Part model, mm, in its own coordinate system. Face numbers are marked on the shaded views. A direction names the side the tool comes from. Coordinates: 2 decimals unless noted, no trailing zeros. Loops run counter-clockwise (first coordinate to the right, second up) from the corner with the lowest first, then second, coordinate; pieces in that order, holes last. Notation, with made-up numbers: (-21.75, 29) -> (-17.75, 29) arc R27 ccw to (-17.75, 48) -> close; hole circle Ø10 at (43, -27). An arc over 180 degrees is marked (long way). Use one line per item in the form item = value. Start each with the question number.
(1) Mould opens along Y. For the marked faces 3, 4, 5 and 6 say: +Y half, -Y half, draft (parallel to the pull), parting line (faces both ways), or undercut.
(2) Band-saw the part on D-D on y = -6. Count the separate pieces of the cut face and the enclosed holes in it, then the cut area to 3 significant figures.
(3) Band-saw the part on A-A on x = 0. Give the cut face in (y, z).
(4) Band-saw the part on B-B on z = -1. Give the cut face in (x, y).
(5) Drill centre lines: L1, parallel to Z at x = -1, y = 0.5; L2, parallel to Z at x = -20, y = 1.75; L3, parallel to Y at x = -21, z = -10.5. Where is each one in solid material? Low to high. Write a range as [from, to].
(6) 3-axis set-ups, long thin cutter, end or side, ignore diameter. For the marked faces 1 and 2: which of +Z, -Z, +X, -X, +Y, -Y reach the whole face in a straight line?
(7) Band-saw the part on C-C on x = -27. Give the cut face in (y, z).
(8) Pin check, flat tips, straight feed: P1, Ø2, axis at x = 0, y = -6, coming from the -Z side; P2, Ø1.7, axis at x = -9.88, y = -6, coming from the -Z side; P3, Ø0.6, axis at y = 0.5, z = -8.5, coming from the -X side; P4, Ø2.5, axis at y = 0, z = 13, coming from the +X side. Stop position of each tip, or through.
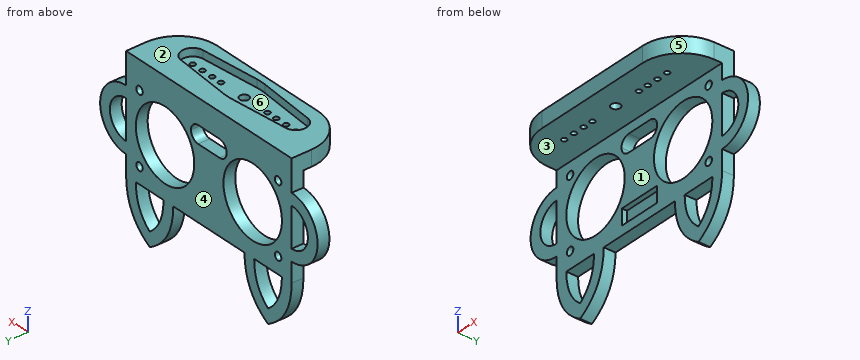
```python
from build123d import *

# Parameters (mm, degrees)
SKETCH1_R           = 1
SKETCH1_R_2         = 9
BOSS_EXTRUDE3_DEPTH = 3
BOSS_EXTRUDE4_DEPTH = 15
SKETCH5_R           = 0.6604
SKETCH5_R_2         = 1.143
CUT_EXTRUDE1_DEPTH  = 10
FILLET2_R           = 10
CUT_EXTRUDE3_DEPTH  = 2
SKETCH8_W           = 10.76
SKETCH8_H           = 4
CUT_EXTRUDE4_DEPTH  = 1.3


with BuildPart() as part:
    # Sketch1 → Boss-Extrude3 (new body)
    with BuildSketch(Plane(origin=(0, 0, 0), x_dir=(1, 0, 0), z_dir=(0, 1, 0))):
        with BuildLine():
            Line((-25.5, -8), (-25.5, -13))
            Line((-25.5, -13), (25.5, -13))
            Line((25.5, -13), (25.5, -8))
            ThreePointArc((25.5, -8), (33.5, 0), (25.5, 8))
            Line((25.5, 8), (25.5, 13))
            add(Edge.make_bspline(
                [(25.5, 13), (25.447957122, 21.830633136), (18.232464907, 26.037260317)],
                knots=[0, 0, 0, 1, 1, 1], degree=2))
            add(Edge.make_bspline(
                [(10.964929815, 13), (11.016972693, 21.830633136), (18.232464907, 26.037260317)],
                knots=[0, 0, 0, 1, 1, 1], degree=2))
            Line((10.964929815, 13), (-10.964929815, 13))
            add(Edge.make_bspline(
                [(-10.964929815, 13), (-11.016972693, 21.830633136), (-18.232464907, 26.037260317)],
                knots=[0, 0, 0, 1, 1, 1], degree=2))
            add(Edge.make_bspline(
                [(-25.5, 13), (-25.447957122, 21.830633136), (-18.232464907, 26.037260317)],
                knots=[0, 0, 0, 1, 1, 1], degree=2))
            Line((-25.5, 13), (-25.5, 8))
            ThreePointArc((-25.5, 8), (-33.5, 0), (-25.5, -8))
        make_face()
        with Locations((-21.330701069, -8.788977071)):
            Circle(SKETCH1_R, mode=Mode.SUBTRACT)
        with BuildLine():
            ThreePointArc((-25.5, -5), (-30.5, 0), (-25.5, 5))
            Line((-25.5, 5), (-25.5, -5))
        make_face(mode=Mode.SUBTRACT)
        with Locations((-13.5, 0)):
            Circle(SKETCH1_R_2, mode=Mode.SUBTRACT)
        with BuildLine():
            ThreePointArc((-5.5, -7.45), (-4.855634919, -5.894365081), (-3.3, -5.25))
            Line((-3.3, -5.25), (3.3, -5.25))
            ThreePointArc((3.3, -5.25), (4.855634919, -5.894365081), (5.5, -7.45))
            ThreePointArc((5.5, -7.45), (4.855634919, -9.005634919), (3.3, -9.65))
            Line((3.3, -9.65), (-3.3, -9.65))
            ThreePointArc((-3.3, -9.65), (-4.855634919, -9.005634919), (-5.5, -7.45))
        make_face(mode=Mode.SUBTRACT)
        with Locations((21.36922293, -8.864067488)):
            Circle(SKETCH1_R, mode=Mode.SUBTRACT)
        with Locations((13.5, 0)):
            Circle(SKETCH1_R_2, mode=Mode.SUBTRACT)
        with BuildLine():
            Line((25.5, -5), (25.5, 5))
            ThreePointArc((25.5, 5), (30.5, 0), (25.5, -5))
        make_face(mode=Mode.SUBTRACT)
        with Locations((-21.330701069, 8.788977071)):
            Circle(SKETCH1_R, mode=Mode.SUBTRACT)
        with BuildLine():
            add(Edge.make_bspline(
                [(-18.232464907, 22.430397358), (-17.881752173, 22.15826664), (-17.197190326, 21.563514811), (-16.070323369, 20.318879343), (-15.204967784, 18.922941442), (-14.583600481, 17.329273987), (-14.239247895, 16.018289812), (-14.058547206, 14.81714331), (-13.98211291, 13.800154377), (-13.966795322, 13.26237878), (-13.964990622, 12.999999994)],
                knots=[0, 0, 0, 0, 0.107910014, 0.215820028, 0.431640056, 0.53955007, 0.647460084, 0.755370098, 0.809325105, 0.862094482, 0.862094482, 0.862094482, 0.862094482], degree=3))
            Line((-13.964990622, 12.999999994), (-22.499939192, 12.999999994))
            add(Edge.make_bspline(
                [(-22.499939192, 12.999999994), (-22.498134493, 13.26237878), (-22.482816904, 13.800154377), (-22.406382608, 14.81714331), (-22.22568192, 16.018289812), (-21.881329334, 17.329273987), (-21.259962031, 18.922941442), (-20.394606445, 20.318879343), (-19.267739489, 21.563514811), (-18.583177642, 22.15826664), (-18.232464907, 22.430397358)],
                knots=[0.00118563, 0.00118563, 0.00118563, 0.00118563, 0.053955007, 0.107910014, 0.215820028, 0.323730042, 0.431640056, 0.647460084, 0.755370098, 0.863280112, 0.863280112, 0.863280112, 0.863280112], degree=3))
        make_face(mode=Mode.SUBTRACT)
        with Locations((21.36922293, 8.864067488)):
            Circle(SKETCH1_R, mode=Mode.SUBTRACT)
        with BuildLine():
            Line((22.499939192, 13), (13.964990622, 13))
            add(Edge.make_bspline(
                [(13.964990622, 13), (13.966795322, 13.262378784), (13.982112911, 13.800154379), (14.058547206, 14.81714331), (14.239247895, 16.018289812), (14.583600481, 17.329273987), (15.204967784, 18.922941442), (16.070323369, 20.318879343), (17.197190326, 21.563514811), (17.881752173, 22.15826664), (18.232464907, 22.430397358)],
                knots=[0.00118563, 0.00118563, 0.00118563, 0.00118563, 0.053955007, 0.107910014, 0.215820028, 0.323730042, 0.431640056, 0.647460084, 0.755370098, 0.863280112, 0.863280112, 0.863280112, 0.863280112], degree=3))
            add(Edge.make_bspline(
                [(18.232464907, 22.430397358), (18.583177642, 22.15826664), (19.267739489, 21.563514811), (20.394606445, 20.318879343), (21.259962031, 18.922941442), (21.881329334, 17.329273987), (22.22568192, 16.018289812), (22.406382608, 14.81714331), (22.482816904, 13.800154379), (22.498134493, 13.262378784), (22.499939192, 13)],
                knots=[0, 0, 0, 0, 0.107910014, 0.215820028, 0.431640056, 0.53955007, 0.647460084, 0.755370098, 0.809325105, 0.862094482, 0.862094482, 0.862094482, 0.862094482], degree=3))
        make_face(mode=Mode.SUBTRACT)
    extrude(amount=BOSS_EXTRUDE3_DEPTH)

    # Sketch4 → Boss-Extrude4 (add)
    with BuildSketch(Plane(origin=(0, 3, 0), x_dir=(1, 0, 0), z_dir=(0, 1, 0))):
        Polygon((-25.5, -13), (-25.5, -16), (25.5, -16), (25.5, -13), (25.5, -12), (-25.5, -12), align=None)
    extrude(amount=-BOSS_EXTRUDE4_DEPTH)

    # Sketch5 → Cut-Extrude1 (cut)
    with BuildSketch(Plane(origin=(0, 0, 12), x_dir=(-1, 0, 0), z_dir=(0, 0, -1))):
        with Locations((-15.875, -6)):
            Circle(SKETCH5_R)
        with Locations((-12.8778, -6)):
            Circle(SKETCH5_R)
        with Locations((-9.8806, -6)):
            Circle(SKETCH5_R)
        with Locations((-7.1628, -6)):
            Circle(SKETCH5_R)
        with Locations((15.875, -6)):
            Circle(SKETCH5_R)
        with Locations((12.8778, -6)):
            Circle(SKETCH5_R)
        with Locations((9.8806, -6)):
            Circle(SKETCH5_R)
        with Locations((7.1628, -6)):
            Circle(SKETCH5_R)
        with Locations((0, -6)):
            Circle(SKETCH5_R_2)
    extrude(amount=-CUT_EXTRUDE1_DEPTH, mode=Mode.SUBTRACT)

    # Fillet2
    fillet2_edges = [part.edges().sort_by_distance(p)[0] for p in [
        (25.5, -12, 14),
        (-25.5, -12, 14),
    ]]
    fillet(fillet2_edges, radius=FILLET2_R)

    # Sketch7 → Cut-Extrude3 (cut)
    with BuildSketch(Plane.XY.offset(16)):
        with BuildLine():
            Line((1.237363975, -10.208408252), (16.139135026, -8.805342715))
            ThreePointArc((16.139135026, -8.805342715), (18.69275, -6), (16.139135026, -3.194657285))
            Line((16.139135026, -3.194657285), (1.237363975, -1.791591748))
            ThreePointArc((1.237363975, -1.791591748), (0, -1.733468722), (-1.237363975, -1.791591748))
            Line((-1.237363975, -1.791591748), (-16.139135026, -3.194657285))
            ThreePointArc((-16.139135026, -3.194657285), (-18.69275, -6), (-16.139135026, -8.805342715))
            Line((-16.139135026, -8.805342715), (-1.237363975, -10.208408252))
            ThreePointArc((-1.237363975, -10.208408252), (0, -10.266531278), (1.237363975, -10.208408252))
        make_face()
    extrude(amount=-CUT_EXTRUDE3_DEPTH, mode=Mode.SUBTRACT)

    # Sketch8 → Cut-Extrude4 (cut)
    with BuildSketch(Plane.XZ):
        with Locations((0, -8.7)):
            Rectangle(SKETCH8_W, SKETCH8_H)
    extrude(amount=-CUT_EXTRUDE4_DEPTH, mode=Mode.SUBTRACT)


solid = part.part
```
A:
q1.face_3 = draft
q1.face_4 = +Y half
q1.face_5 = -Y half
q1.face_6 = undercut
q2.separate_pieces = 10
q2.enclosed_holes = 0
q2.area = 96.8 mm²
q3.outline = (-12, 12) -> (-7.14, 12) -> (-7.14, 14) -> (-10.27, 14) -> (-10.27, 16) -> (-12, 16) -> close; (-4.86, 12) -> (0, 12) -> (0, 9.65) -> (3, 9.65) -> (3, 16) -> (-1.73, 16) -> (-1.73, 14) -> (-4.86, 14) -> close; (0, -13) -> (3, -13) -> (3, 5.25) -> (0, 5.25) -> (0, -6.7) -> (1.3, -6.7) -> (1.3, -10.7) -> (0, -10.7) -> close
q4.outline = (-33.44, 0) -> (-30.4, 0) -> (-30.4, 3) -> (-33.44, 3) -> close; (-25.5, 0) -> (-22.44, 0) -> (-22.44, 3) -> (-25.5, 3) -> close; (-4.56, 0) -> (4.56, 0) -> (4.56, 3) -> (-4.56, 3) -> close; (22.44, 0) -> (25.5, 0) -> (25.5, 3) -> (22.44, 3) -> close; (30.4, 0) -> (33.44, 0) -> (33.44, 3) -> (30.4, 3) -> close
q5.L1 = [-13, -10.7], [-6.7, 5.25], [9.65, 16]
q5.L2 = [-24.86, -20.73], [-13, -6.22], [6.22, 16]
q5.L3 = [0, 3]
q6.face_1 = -Z, +X, -X, -Y
q6.face_2 = +Z, +X, -X, +Y, -Y
q7.outline = (0, -7.86) -> (3, -7.86) -> (3, -4.77) -> (0, -4.77) -> close; (0, 4.77) -> (3, 4.77) -> (3, 7.86) -> (0, 7.86) -> close
q8.P1 = through
q8.P2 = 12
q8.P3 = -25.5
q8.P4 = 25.5
